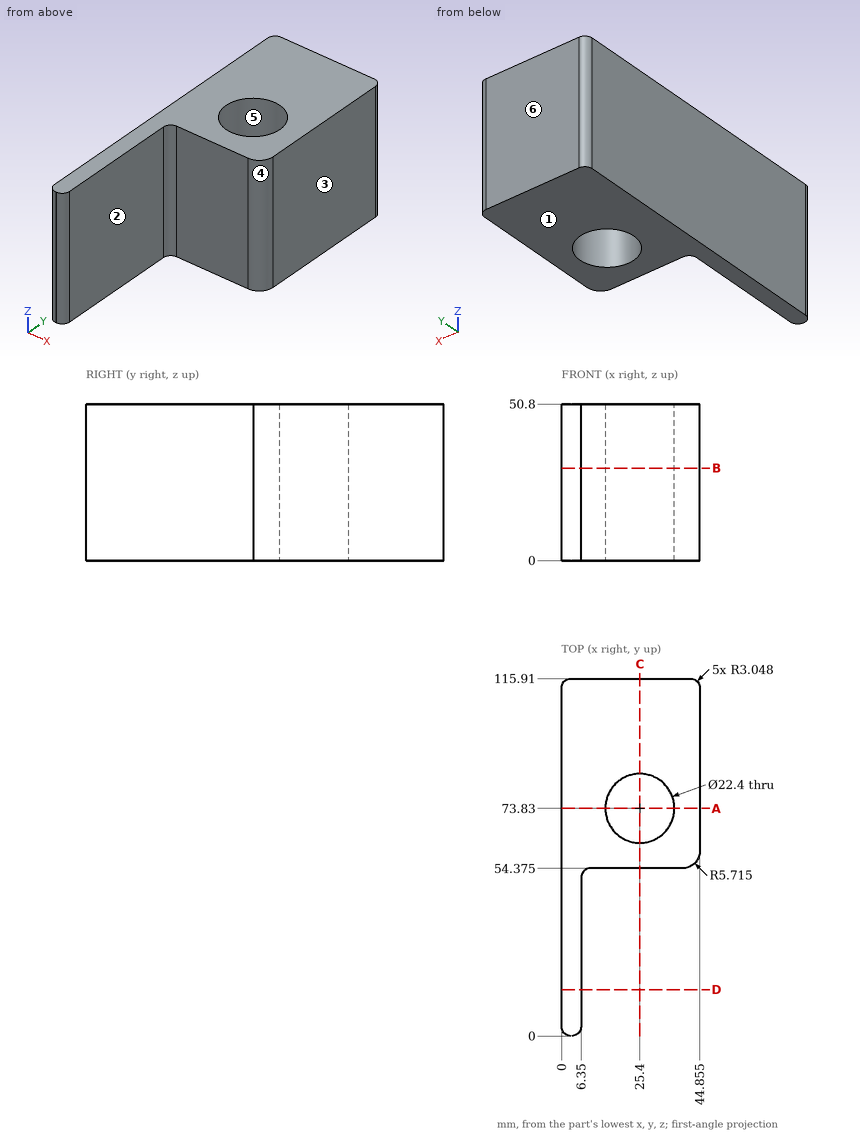
Verification items for this drawing (mm, ordinates from the low corner). A direction names the side the tool comes from. Give positions to 0.01 mm unless a question says otherwise; leave off trailing zeros. Loops run counter-clockwise (first coordinate to the right, second up) from the corner with the lowest first, then second, coordinate; pieces in that order, holes last. Notation, with made-up numbers: M 80.5,66 L 109.5,66 A33 ccw 109.5,104 Z; hole C -34,-22.75 d10. An arc over 180 degrees is marked long. Write each question's results on one line, items separated by ' | '.
1) Section check B-B, the plane z = 30. Record the boundary of the cut face in (x, y) (3 decimals), plus the area to 3 significant figures.
Answers follow:
outline: M 0,3.048 A3.048 ccw 3.048,0 L 3.302,0 A3.048 ccw 6.35,3.048 L 6.35,51.327 A3.048 cw 9.398,54.375 L 39.14,54.375 A5.715 ccw 44.855,60.09 L 44.855,112.862 A3.048 ccw 41.807,115.91 L 3.048,115.91 A3.048 ccw 0,112.862 Z; hole C 25.4,73.83 d22.4 | area: 2,700 mm2
2) Gauge pin test, flat ends, axial feed: pin 1 (5 mm diameter, centred on x = 39, y = 94, fed in from -Z); pin 2 (1.5 mm diameter, centred on x = 8.5, z = 44, fed in from -Y); pin 3 (1.5 mm diameter, centred on y = 57, z = 8, fed in from +X); pin 4 (6 mm diameter, centred on x = 22, z = 35.5, fed in from -Y) (3 decimals). Record the tip position at first contact, or that the pin passes through.
Answers follow:
pin 1: z = 0 | pin 2: y = 53.89 | pin 3: x = 44.35 | pin 4: y = 54.375
3) Section check A-A, the plane y = 73.83. Record the boundary of the cut face in (x, z) (3 decimals), plus the area to 3 significant figures.
Answers follow:
outline: M 0,0 L 14.2,0 L 14.2,50.8 L 0,50.8 Z; M 36.6,0 L 44.855,0 L 44.855,50.8 L 36.6,50.8 Z | area: 1,140 mm2
4) Section check C-C, the plane x = 25.4. Record the boundary of the cut face in (y, z) (3 decimals).
Answers follow:
outline: M 54.375,0 L 62.63,0 L 62.63,50.8 L 54.375,50.8 Z; M 85.03,0 L 115.91,0 L 115.91,50.8 L 85.03,50.8 Z
5) Thickness scan on line 1 (X direction, y = 73.83, z = 15.5) (3 decimals); line 2 (Y direction, x = 25.4, z = 23) (3 decimals); line 3 (X direction, y = 10.5, z = 25). Record the ranges inside material, lowest first.
Answers follow:
line 1: 0 to 14.2, 36.6 to 44.855 | line 2: 54.375 to 62.63, 85.03 to 115.91 | line 3: 0 to 6.35
6) Section check D-D, the plane y = 15. Record the boundary of the cut face in (x, z), plus the area to 3 significant figures.
Answers follow:
outline: M 0,0 L 6.35,0 L 6.35,50.8 L 0,50.8 Z | area: 323 mm2
7) Release check for a two-part mould opening along Y. For the marked faces 3, 4, 5 and 6 record: +Y half, -Y half, draft (parallel to the pull), parting line (faces both ways), or undercut.
Answers follow:
face 3: draft | face 4: -Y half | face 5: undercut | face 6: +Y half
8) Tool access check on the marked faces 1 and 2. Record the directions out of +Z, -Z, +X, -X, +Y, -Y that give a thin tool (end or side, any length) a straight path to the whole face; none if there is none.
Answers follow:
face 1: -Z, +X, -X, +Y, -Y | face 2: +Z, -Z, +X, -Y
